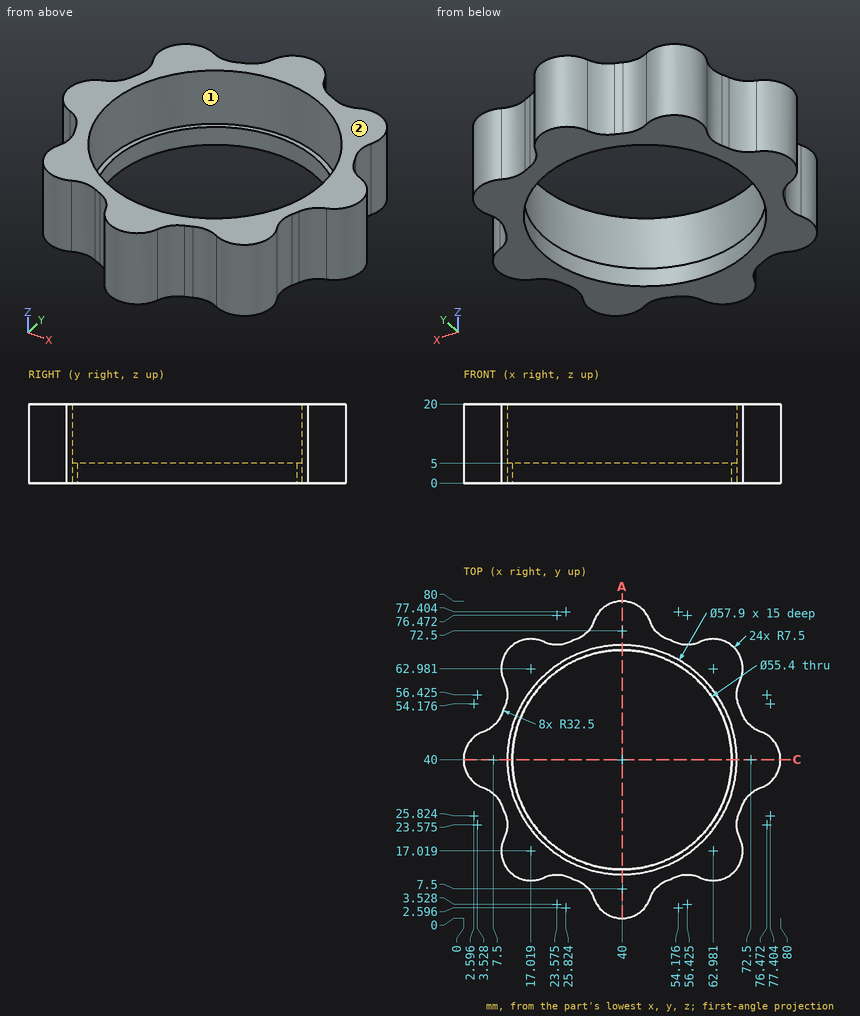
Drawing for the job (mm, zero at the part's lowest x, y, z). Give positions to 0.01 mm unless a question says otherwise; leave off trailing zeros. Order: outer loops, then holes, each group sorted by start corner. A loop starts at its lowest first (then second) coordinate and runs counter-clockwise, first axis right, second up. Notation, with made-up numbers: M -5,-14.75 L 3,-14.75 A8 ccw 3,0.25 Z; hole C 46.5,14 d1. An arc over 180 degrees is marked long. Write item = value, one per line. Start each with the question number.
(1) Two-plate mould, pull along X, no slides. Class the marked faces 1 and 2: released by +X, released by -X, zero draft, split by the parting line, or undercut.
(2) Slice it at A-A on x = 40. Write the cut outline in (y, z).
(3) Probe L1, parallel to Y at x = 40, z = 1.9; L2, parallel to Y at x = 20, z = 10. List the from-to ranges inside material, lowest first. Write a range as [from, to].
(4) Pin check, flat tips, straight feed: pin 1 Ø10 at (y, z) = (52.5, 6.5) entering from +X (1 decimal); pin 2 Ø6 at (y, z) = (36, 8) entering from -X; pin 3 Ø5 at (x, z) = (11.5, 6.5) entering from +Y. Stop position of each tip, or through.
Responses:
q1.face_1 = undercut
q1.face_2 = zero draft
q2.outline = M 0,0 L 12.3,0 L 12.3,5 L 11.05,5 L 11.05,20 L 0,20 Z; M 67.7,0 L 80,0 L 80,20 L 68.95,20 L 68.95,5 L 67.7,5 Z
q3.L1 = [0, 12.3], [67.7, 80]
q3.L2 = [10.14, 19.07], [60.93, 69.86]
q4.pin_1 = 74
q4.pin_2 = 0.07
q4.pin_3 = 69.85
